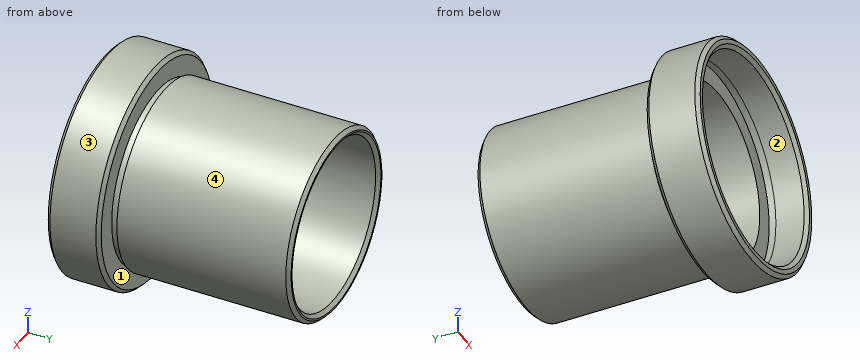
```python
from build123d import *


with BuildPart() as part:
    # 草图1 → 旋转2 (revolve)
    with BuildSketch(Plane.XY, mode=Mode.PRIVATE) as revolve_2_sk:
        Polygon((12.25, 27.042854175), (12.5, 27.042854175), (13, 26.542854175), (13, 2.642854175), (12.5, 2.642854175), (12.5, 1.642854175), (15.375, 1.642854175), (15.875, 1.142854175), (15.875, -5.357145825), (15.375, -5.857145825), (14.75, -5.857145825), (14.25, -5.357145825), (14.25, -1.357145825), (14.35, -1.357145825), (14.35, -0.357145825), (11.75, -0.357145825), (11.75, 26.542854175), align=None)
    revolve(revolve_2_sk.sketch.rotate(Axis((0, 44.598597745, 0), (0, -1, 0)), 90), axis=Axis((0, 44.598597745, 0), (0, -1, 0)))  # turned: the seam where the file's is


solid = part.part
```
Input: part model. Units: mm. Frame: model coordinates. Face numbers are marked on the shaded views. A direction names the side the tool comes from. Round coordinates to 2 decimals unless told otherwise and drop trailing zeros. Loops run counter-clockwise (first coordinate to the right, second up) from the corner with the lowest first, then second, coordinate; pieces in that order, holes last. Notation, with made-up numbers: (-20.5, 27) -> (-6.5, 27) arc R19 ccw to (-6.5, 47) -> close; hole circle Ø5 at (58.5, 11). An arc over 180 degrees is marked (long way). Use one line per item in the form item = value. Start each with the question number.
Item 1: Section query C-C on y = 14.5. Return the cut outline in (x, z), then the cut area to 3 significant figures.
Item 2: Set-up query: the marked faces 1, 2, 3 and 4. Return all of +Z, -Z, +X, -X, +Y, -Y with unobstructed straight access to the full face (end or side cutting, diameter ignored); none if empty.
Item 3: Contact query for flat-ended pins moving along their axis: pin 1 Ø13 at (x, z) = (-4.5, -3.5) entering from -Y; pin 2 Ø1 at (x, y) = (-9.5, 23) entering from +Z; pin 3 Ø12 at (x, y) = (8.5, 20) entering from -Z. Output: stop coordinate, or through.
Item 4: Material intervals for L1, parallel to X at y = 21, z = 0; L2, parallel to Z at x = -4, y = 21; L3, parallel to X at y = -3.1, z = 0 (3 decimals), sorted ascending. Write a range as from..to.
Ans:
q1.outline = circle Ø26 at (0, 0); hole circle Ø23.5 at (0, 0)
q1.area = 97.2 mm^2
q2.face_1 = none
q2.face_2 = -Y
q2.face_3 = +Y, -Y
q2.face_4 = +Y
q3.pin_1 = -0.36
q3.pin_2 = 9.38
q3.pin_3 = -12.76
q4.L1 = -13..-11.75, 11.75..13
q4.L2 = -12.37..-11.05, 11.05..12.37
q4.L3 = -15.875..-14.25, 14.25..15.875
